```python
from build123d import *

# Parameters (mm, degrees)
BOSS_EXTRUDE1_DEPTH = 5.08
SKETCH2_W           = 25.4
SKETCH2_H           = 25.4
CUT_EXTRUDE1_DEPTH  = 206.587072794


with BuildPart() as part:
    # Sketch1 → Boss-Extrude1 (new body)
    with BuildSketch(Plane.XY):
        Polygon((0, 0), (0, -20.602222222), (-5.08, -20.602222222), (-5.08, -41.204444444), (0, -41.204444444), (0, -61.806666667), (-5.08, -61.806666667), (-5.08, -82.408888889), (0, -82.408888889), (0, -103.011111111), (-5.08, -103.011111111), (-5.08, -123.613333333), (0, -123.613333333), (0, -144.215555556), (-5.08, -144.215555556), (-5.08, -164.817777778), (0, -164.817777778), (0, -185.42), (6.35, -185.42), (6.35, -200.66), (19.05, -200.66), (19.05, -185.42), (22.225, -185.42), (22.225, -156.21), (44.45, -156.21), (44.45, -29.21), (22.225, -29.21), (22.225, 0), (19.05, 0), (19.05, 15.24), (6.35, 15.24), (6.35, 0), align=None)
    extrude(amount=BOSS_EXTRUDE1_DEPTH)

    # Sketch2 → Cut-Extrude1 (cut, through all)
    with BuildSketch(Plane.XY.offset(5.08)):
        with Locations((44.45, -92.71)):
            Rectangle(SKETCH2_W, SKETCH2_H)
    extrude(amount=-CUT_EXTRUDE1_DEPTH, mode=Mode.SUBTRACT)


solid = part.part
```
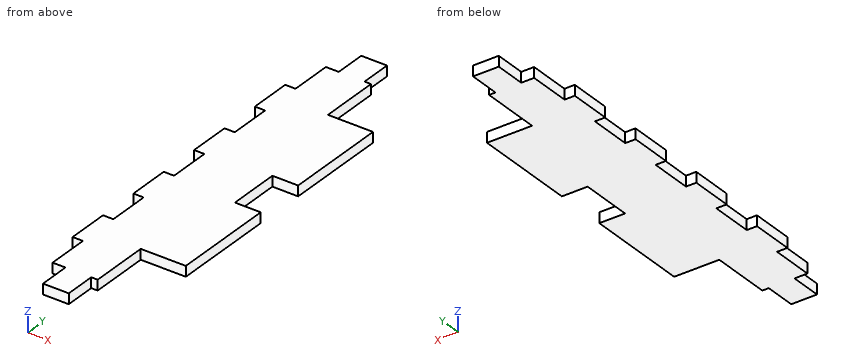
The model under review builds one solid part; all positions refer to its coordinate system, in mm. Round coordinates to 2 decimals unless told otherwise and drop trailing zeros. Order: outer loops, then holes, each group sorted by start corner. A loop starts at its lowest first (then second) coordinate and runs counter-clockwise, first axis right, second up. Notation, with made-up numbers: (78.25, 18.25) - (84.25, 18.25) arc R20 cw to (84.25, 23.25) - close; hole circle Ø4 at (15.25, -12). An arc over 180 degrees is marked (long way). Answer in a Markdown table with one row per item.
(1) Take a section at C-C on x = 4.5. Write out the cut boundary in (y, z).
Result set:
| item | result |
|---|---|
| outline | (-185.42, 0) - (0, 0) - (0, 5.08) - (-185.42, 5.08) - close |
(2) Take a section at A-A on x = 37.5. Write out the cut boundary in (y, z).
Result set:
| item | result |
|---|---|
| outline | (-156.21, 0) - (-105.41, 0) - (-105.41, 5.08) - (-156.21, 5.08) - close; (-80.01, 0) - (-29.21, 0) - (-29.21, 5.08) - (-80.01, 5.08) - close |
(3) Clearance check with flat-ended pins moving along their axes: P1, Ø1.5, axis at x = -1.5, z = 3, coming from the -Y side; P2, Ø1.5, axis at y = 5.5, z = 3.5, coming from the +X side; P3, Ø1.5, axis at y = -86.5, z = 1.5, coming from the +X side. State where each tip first meets the part, or that it passes through.
Result set:
| item | result |
|---|---|
| P1 | stops at y = -164.82 |
| P2 | stops at x = 19.05 |
| P3 | stops at x = 31.75 |
(4) Take a section at B-B on y = -167.5. Write out the cut boundary in (x, z) (3 decimals).
Result set:
| item | result |
|---|---|
| outline | (0, 0) - (22.225, 0) - (22.225, 5.08) - (0, 5.08) - close |
(5) For line 1 (Y direction, x = -1.5, z = 3.65); line 2 (Y direction, x = 41.5, z = 4.65); line 3 (X direction, y = -129, z = 0.35), list the stretches that pass through material, from the lowest coordinate up. Write a range as from..to.
Result set:
| item | result |
|---|---|
| line 1 | y = -164.82..-144.22, -123.61..-103.01, -82.41..-61.81, -41.2..-20.6 |
| line 2 | y = -156.21..-105.41, -80.01..-29.21 |
| line 3 | x = 0..44.45 |
